Autodesk Inventor part; units mm, degrees
ref_plane "YZ Plane" through (0, 0, 0) normal (1, 0, 0) x (0, 1, 0)
ref_plane "XZ Plane" through (0, 0, 0) normal (0, 1, 0) x (-1, 0, 0)
ref_plane "XY Plane" through (0, 0, 0) normal (0, 0, 1) x (1, 0, 0)
sketch "Sketch1" plane through (0, 0, 0) normal (1, 0, 0) x (0, 1, 0)
  line L0 (32.5, 9) -> (-32.5, 9)
  line L1 (-32.5, 9) -> (-32.5, -9)
  line L2 (-32.5, -9) -> (32.5, -9)
  line L3 (32.5, -9) -> (32.5, 9)
  line L4 (32.5, 9) -> (-32.5, -9) construction
  line L5 (-32.5, 9) -> (32.5, -9) construction
  circle A0 centre (-25, 0) radius 3
  circle A1 centre (25, 0) radius 3
  line L6 (-3, -5) -> (-3, 5) construction
  line L7 (-6, -5) -> (-6, 5)
  line L8 (0, 5) -> (0, -5)
  arc A2 (-6, -5) -> (0, -5) centre (-3, -5) ccw
  arc A3 (0, 5) -> (-6, 5) centre (-3, 5) ccw
  line L9 (17, -5) -> (17, 5) construction
  line L10 (20, -5) -> (20, 5)
  line L11 (14, 5) -> (14, -5)
  arc A4 (14, -5) -> (20, -5) centre (17, -5) ccw
  arc A5 (20, 5) -> (14, 5) centre (17, 5) ccw
  point P0 (0, 0)
  point P1 (-3, 0)
  point P2 (17, 0)
  point P3 (0, 0)
  dimension "d0" = 25
  dimension "d1" = 50
  dimension "d2" = 65
  dimension "d3" = 6
  dimension "d5" = 20
  dimension "d6" = 10
  dimension "d7" = 3
  dimension "d8" = 18
  dimension "d36" = 3
extrude "Extrusion1" add sketch "Sketch1" along normal blind 12
sketch "Sketch2" plane through (0, 0, 0) normal (-1, 0, 0) x (0, 0, 1)
  line L0 (9, -32.5) -> (-9, -32.5)
  line L1 (9, 32.5) -> (9, -32.5)
  line L2 (-9, 32.5) -> (9, 32.5)
  line L3 (-9, -32.5) -> (-9, 32.5)
  circle A0 centre (0, -25) radius 3
  circle A1 centre (0, 25) radius 3
  arc A2 (-5, 20) -> (-5, 14) centre (-5, 17) ccw
  line L4 (5, 20) -> (-5, 20)
  arc A3 (5, 14) -> (5, 20) centre (5, 17) ccw
  line L5 (-5, 14) -> (5, 14)
  line L6 (5, 0) -> (-5, 0)
  arc A4 (5, -6) -> (5, 0) centre (5, -3) ccw
  line L7 (-5, -6) -> (5, -6)
  arc A5 (-5, 0) -> (-5, -6) centre (-5, -3) ccw
  line L8 (5, 17) -> (-5, 17) construction
  line L9 (5, 15.25) -> (-5, 15.25)
  line L10 (-5, 18.75) -> (5, 18.75)
  arc A6 (5, 15.25) -> (5, 18.75) centre (5, 17) ccw
  arc A7 (-5, 18.75) -> (-5, 15.25) centre (-5, 17) ccw
  line L11 (5, -3) -> (-5, -3) construction
  line L12 (5, -4.75) -> (-5, -4.75)
  line L13 (-5, -1.25) -> (5, -1.25)
  arc A8 (5, -4.75) -> (5, -1.25) centre (5, -3) ccw
  arc A9 (-5, -1.25) -> (-5, -4.75) centre (-5, -3) ccw
  point P0 (0, 0)
  point P1 (0, 17)
  point P2 (0, -3)
  dimension "d11" = 3.5
extrude "Extrusion2" add sketch "Sketch2" against normal blind 3 contours L4 A3 L5 A2 | A4 L7 A5 L6
chamfer "Chamfer1" distance 5 angle 45 4 edges at (6, -32.5, 9) (6, -32.5, -9) (6, 32.5, -9) (6, 32.5, 9)
sketch "Sketch3" plane through (0, -27.5, 9) normal (0, 0, 1) x (1, 0, 0)
  line L0 (0, 55) -> (12, 55)
  line L1 (0, 55) -> (0, 0)
  line L2 (12, 0) -> (0, 0)
  line L3 (12, 55) -> (12, 0)
  line L4 (12, 10) -> (8.5, 10)
  line L5 (8.5, 10) -> (8.5, 45)
  line L6 (8.5, 45) -> (12, 45)
  line L7 (12, 45) -> (12, 10)
  line L8 (12, 10) -> (8.5, 45) construction
  line L9 (8.5, 10) -> (12, 45) construction
  point P0 (0, 27.5)
  point P1 (10.25, 27.5)
  point P2 (0, 27.5)
  point P3 (12, 10)
  dimension "d17" = 35
  dimension "d18" = 3.5
extrude "Extrusion3" cut sketch "Sketch3" against normal through all contours L3 L4 L5 L6
equation "\"d1\" = 2 * d0"
properties part number "ToolDock_R" material "PET Plastic"
The listing builds one solid part. Answer for the finished solid, in the listing's coordinates (mm). A direction names the side the tool comes from. Give positions to 0.01 mm unless a question says otherwise; leave off trailing zeros. Loops run counter-clockwise (first coordinate to the right, second up) from the corner with the lowest first, then second, coordinate; pieces in that order, holes last. Notation, with made-up numbers: (-40, -39.5) - (-19, -39.5) arc R10 ccw to (-19, -27.5) - close; hole circle Ø7 at (82.25, 79.5). An arc over 180 degrees is marked (long way). Answer as a JSON object with one key per item and string values.
1. A cutting plane is placed at A-A (z = 0). Give the number of separate pieces and of enclosed holes in the cut face, then the cut area to 3 significant figures.
Determined:
{"separate pieces": "5", "enclosed holes": "0", "area": "418 mm²"}
2. Find the intervals of material crossed by L1, parallel to Y at x = 4.25, z = -6.25; L2, parallel to Z at x = 3.5, y = 17; L3, parallel to Y at x = 10, z = -3.25, in increasing order. Write a range as [from, to].
Determined:
{"L1": "[-30.25, -5.73], [-0.27, 14.27], [19.73, 30.25]", "L2": "[-9, -8], [8, 9]", "L3": "[-32.5, -17.5], [20, 32.5]"}
3. A cutting plane is placed at D-D (z = 5.75). Write down the section's boundary in (x, y), then the cut area to 3 significant figures.
Determined:
{"outline": "(0, -30.75) - (12, -30.75) - (12, -17.5) - (8.5, -17.5) - (8.5, -5.9) - (3, -5.9) - (3, -4.58) - (0, -4.58) - close; (0, -1.42) - (3, -1.42) - (3, -0.1) - (8.5, -0.1) - (8.5, 14.1) - (3, 14.1) - (3, 15.42) - (0, 15.42) - close; (0, 18.58) - (3, 18.58) - (3, 19.9) - (12, 19.9) - (12, 30.75) - (0, 30.75) - close", "area": "524 mm²"}
4. For a pull along Y with two mould halves and no side action, classify faces 1 (the flat face through (6.1, -30, 6.5)), 2 (the flat face through (3, -5, 0)), 3 (the flat face through (12, -21.8, 0.1)) as pulls with the +Y half, pulls with the -Y half, needs draft (parallel to the pull), parting line crosses it, or undercut.
Determined:
{"face 1": "pulls with the -Y half", "face 2": "undercut", "face 3": "needs draft"}
5. For faces 4 (the cylindrical face through (1.48, -3.04, 6.75)), 5 (the cylindrical face through (6, -3, 8)), 6 (the flat face through (6, -32.5, 0)), 7 (the flat face through (10.2, 17.5, -8.5)), determine the directions among +Z, -Z, +X, -X, +Y, -Y from which every point of the face is accessible in a straight line to the end or side of a thin tool.
Determined:
{"face 4": "+X, -X", "face 5": "+X", "face 6": "+Z, -Z, +X, -X, -Y", "face 7": "+Z, -Z, +X"}
6. A cutting plane is placed at B-B (y = -25). Write down the section's boundary in (x, z).
Determined:
{"outline": "(0, -9) - (12, -9) - (12, -3) - (0, -3) - close; (0, 3) - (12, 3) - (12, 9) - (0, 9) - close"}
7. Flat-ended cylindrical pins translate along their axes: pin 1 Ø6.5 at (y, z) = (18.5, -1.5) entering from +X; pin 2 Ø0.8 at (x, z) = (10.5, -8.5) entering from -Y; pin 3 Ø0.5 at (x, z) = (9.5, 8.5) entering from -Y. Find the tip coordinate at first contact, or state that the pin passes through.
Determined:
{"pin 1": "x = 12", "pin 2": "y = -28.4", "pin 3": "y = -28.25"}
8. A cutting plane is placed at C-C (x = 1.25). Write down the section's boundary in (y, z).
Determined:
{"outline": "(-32.5, -4) - (-27.5, -9) - (27.5, -9) - (32.5, -4) - (32.5, 4) - (27.5, 9) - (-27.5, 9) - (-32.5, 4) - close; hole circle Ø6 at (-25, 0); hole (-4.75, -5) arc R1.75 ccw to (-1.25, -5) - (-1.25, 5) arc R1.75 ccw to (-4.75, 5) - close; hole (15.25, -5) arc R1.75 ccw to (18.75, -5) - (18.75, 5) arc R1.75 ccw to (15.25, 5) - close; hole circle Ø6 at (25, 0)"}
